```python
from build123d import *

# Parameters (mm, degrees)
F1_DEPTH = 12.7


with BuildPart() as f1:
    # F0 (on Top) → F1 (new body)
    with BuildSketch(Plane.XY):
        with BuildLine():
            ThreePointArc((-26.2838029012, 5.9890534429), (-24.6151248103, 5.9761621536), (-22.9531423273, 6.1260520558))
            ThreePointArc((-22.9531423273, 6.1260520558), (-49.4660776258, 0.5846286719), (-23.509406267, -7.1545136085))
            ThreePointArc((-23.509406267, -7.1545136085), (-25.4282077221, -7.135411063), (-27.3341276607, -7.3581959791))
            ThreePointArc((-27.3341276607, -7.3581959791), (-46.4726203609, 0.8628055089), (-26.2838029012, 5.9890534429))
        make_face()
        with BuildLine():
            Line((-24.5101160102, 0), (-21.5383160102, 0))
            ThreePointArc((-21.5383160102, 0), (-21.8966174323, 3.1436542152), (-22.9531423273, 6.1260520558))
            ThreePointArc((-22.9531423273, 6.1260520558), (-24.6151248103, 5.9761621536), (-26.2838029012, 5.9890534429))
            ThreePointArc((-26.2838029012, 5.9890534429), (-24.9628562451, 3.1230884685), (-24.5101160102, 0))
        make_face()
        with BuildLine():
            ThreePointArc((-23.509406267, -7.1545136085), (-22.0401002948, -3.7105343879), (-21.5383160102, 0))
            Line((-21.5383160102, 0), (-24.5101160102, 0))
            ThreePointArc((-24.5101160102, 0), (-25.2403619408, -3.9407515105), (-27.3341276607, -7.3581959791))
            ThreePointArc((-27.3341276607, -7.3581959791), (-25.4282077221, -7.135411063), (-23.509406267, -7.1545136085))
        make_face()
        with BuildLine():
            ThreePointArc((-13.97, 0), (-9.8782817332, 9.8782817332), (0, 13.97))
            Line((0, 13.97), (0, 21.2281967688))
            ThreePointArc((0, 21.2281967688), (-4.3381640986, 21.9188431605), (-8.2473894167, 23.922494227))
            ThreePointArc((-8.2473894167, 23.922494227), (-12.1416726615, 12.1663301502), (-22.9531423273, 6.1260520558))
            ThreePointArc((-22.9531423273, 6.1260520558), (-21.8966174323, 3.1436542152), (-21.5383160102, 0))
            Line((-21.5383160102, 0), (-13.97, 0))
        make_face()
        with BuildLine():
            Line((0, -16.5764547127), (0, -13.97))
            ThreePointArc((0, -13.97), (-9.8782817332, -9.8782817332), (-13.97, 0))
            Line((-13.97, 0), (-21.5383160102, 0))
            ThreePointArc((-21.5383160102, 0), (-22.0401002948, -3.7105343879), (-23.509406267, -7.1545136085))
            ThreePointArc((-23.509406267, -7.1545136085), (-14.1800112892, -11.2658599468), (-9.5466303459, -20.3473003831))
            ThreePointArc((-9.5466303459, -20.3473003831), (-5.1321883254, -17.5533202567), (0, -16.5764547127))
        make_face()
        with BuildLine():
            ThreePointArc((13.97, -30.5464547127), (12.8498346481, -25.0653371701), (9.6689764472, -20.4632114615))
            ThreePointArc((9.6689764472, -20.4632114615), (9.263305422, -22.3725482488), (9.0618977051, -24.3140865254))
            ThreePointArc((9.0618977051, -24.3140865254), (10.5029749733, -27.2833396443), (10.9982, -30.5464547127))
            ThreePointArc((10.9982, -30.5464547127), (-2.625018329, -41.2267956255), (-9.7451365483, -25.4481494163))
            ThreePointArc((-9.7451365483, -25.4481494163), (-9.4302368554, -22.9061170685), (-9.5466303459, -20.3473003831))
            ThreePointArc((-9.5466303459, -20.3473003831), (-5.5585283155, -43.3629933627), (13.97, -30.5464547127))
        make_face()
        with BuildLine():
            ThreePointArc((9.6689764472, -20.4632114615), (5.2104698339, -17.5845141131), (0, -16.5764547127))
            Line((0, -16.5764547127), (0, -19.5482547127))
            ThreePointArc((0, -19.5482547127), (5.1193540335, -20.8123590938), (9.0618977051, -24.3140865254))
            ThreePointArc((9.0618977051, -24.3140865254), (9.263305422, -22.3725482488), (9.6689764472, -20.4632114615))
        make_face()
        with BuildLine():
            Line((0, -19.5482547127), (0, -16.5764547127))
            ThreePointArc((0, -16.5764547127), (-5.1321883254, -17.5533202567), (-9.5466303459, -20.3473003831))
            ThreePointArc((-9.5466303459, -20.3473003831), (-9.4302368554, -22.9061170685), (-9.7451365483, -25.4481494163))
            ThreePointArc((-9.7451365483, -25.4481494163), (-5.6959732236, -21.1381449668), (0, -19.5482547127))
        make_face()
        with BuildLine():
            Line((23.0888973165, 0), (13.97, 0))
            ThreePointArc((13.97, 0), (9.8782817332, -9.8782817332), (0, -13.97))
            Line((0, -13.97), (0, -16.5764547127))
            ThreePointArc((0, -16.5764547127), (5.2104698339, -17.5845141131), (9.6689764472, -20.4632114615))
            ThreePointArc((9.6689764472, -20.4632114615), (15.2821696202, -11.4178910111), (24.9617009206, -6.9870408157))
            ThreePointArc((24.9617009206, -6.9870408157), (23.5652185436, -3.6168402197), (23.0888973165, 0))
        make_face()
        with BuildLine():
            ThreePointArc((51.0288973165, 0), (41.7222021913, 13.1686934676), (26.2021990138, 8.7916438716))
            ThreePointArc((26.2021990138, 8.7916438716), (28.5955998519, 8.8133611699), (30.9645498306, 9.1552898349))
            ThreePointArc((30.9645498306, 9.1552898349), (42.2518517126, 9.6950310922), (48.0570973165, 0))
            ThreePointArc((48.0570973165, 0), (40.6825557587, -10.3840985518), (28.4485245075, -6.8426517763))
            ThreePointArc((28.4485245075, -6.8426517763), (26.701686584, -6.8321093301), (24.9617009206, -6.9870408157))
            ThreePointArc((24.9617009206, -6.9870408157), (40.6757375362, -13.4936787729), (51.0288973165, 0))
        make_face()
        with BuildLine():
            ThreePointArc((26.2021990138, 8.7916438716), (23.8902038488, 4.6633048748), (23.0888973165, 0))
            Line((23.0888973165, 0), (26.0606973165, 0))
            ThreePointArc((26.0606973165, 0), (27.3638662242, 5.1929543961), (30.9645498306, 9.1552898349))
            ThreePointArc((30.9645498306, 9.1552898349), (28.5955998519, 8.8133611699), (26.2021990138, 8.7916438716))
        make_face()
        with BuildLine():
            Line((26.0606973165, 0), (23.0888973165, 0))
            ThreePointArc((23.0888973165, 0), (23.5652185436, -3.6168402197), (24.9617009206, -6.9870408157))
            ThreePointArc((24.9617009206, -6.9870408157), (26.701686584, -6.8321093301), (28.4485245075, -6.8426517763))
            ThreePointArc((28.4485245075, -6.8426517763), (26.6747987646, -3.6236584423), (26.0606973165, 0))
        make_face()
        with BuildLine():
            ThreePointArc((0, 13.97), (9.8782817332, 9.8782817332), (13.97, 0))
            Line((13.97, 0), (23.0888973165, 0))
            ThreePointArc((23.0888973165, 0), (23.8902038488, 4.6633048748), (26.2021990138, 8.7916438716))
            ThreePointArc((26.2021990138, 8.7916438716), (14.8492633775, 13.7645914435), (9.476547394, 24.9338921412))
            ThreePointArc((9.476547394, 24.9338921412), (5.0876597937, 22.1875619716), (0, 21.2281967688))
            Line((0, 21.2281967688), (0, 13.97))
        make_face()
        with BuildLine():
            ThreePointArc((13.97, 35.1981967688), (-6.3223757342, 47.655663007), (-8.2473894167, 23.922494227))
            ThreePointArc((-8.2473894167, 23.922494227), (-8.7065761615, 27.0814291625), (-9.7451365483, 30.0998914723))
            ThreePointArc((-9.7451365483, 30.0998914723), (-2.625018329, 45.8785376815), (10.9982, 35.1981967688))
            ThreePointArc((10.9982, 35.1981967688), (10.6803409127, 32.5731784398), (9.7451365483, 30.0998914723))
            ThreePointArc((9.7451365483, 30.0998914723), (9.4225906062, 27.5266793177), (9.476547394, 24.9338921412))
            ThreePointArc((9.476547394, 24.9338921412), (12.7974268331, 29.5958074167), (13.97, 35.1981967688))
        make_face()
        with BuildLine():
            Line((0, 24.1999967688), (0, 21.2281967688))
            ThreePointArc((0, 21.2281967688), (5.0876597937, 22.1875619716), (9.476547394, 24.9338921412))
            ThreePointArc((9.476547394, 24.9338921412), (9.4225906062, 27.5266793177), (9.7451365483, 30.0998914723))
            ThreePointArc((9.7451365483, 30.0998914723), (5.6959732236, 25.7898870228), (0, 24.1999967688))
        make_face()
        with BuildLine():
            ThreePointArc((-8.2473894167, 23.922494227), (-4.3381640986, 21.9188431605), (0, 21.2281967688))
            Line((0, 21.2281967688), (0, 24.1999967688))
            ThreePointArc((0, 24.1999967688), (-5.6959732236, 25.7898870228), (-9.7451365483, 30.0998914723))
            ThreePointArc((-9.7451365483, 30.0998914723), (-8.7065761615, 27.0814291625), (-8.2473894167, 23.922494227))
        make_face()
    extrude(amount=F1_DEPTH)


solid = f1.part
```
Could you check a few things on this model? Use its own coordinates, in mm. A direction names the side the tool comes from. Round coordinates to 2 decimals unless told otherwise and drop trailing zeros. Loops run counter-clockwise (first coordinate to the right, second up) from the corner with the lowest first, then second, coordinate; pieces in that order, holes last. Notation, with made-up numbers: M 58.25,88.25 L 66.25,88.25 A22 ccw 66.25,98.25 Z; hole C 68.5,-13.75 d10. An arc over 180 degrees is marked long. Answer as CSV lines item,"result".
1) We'd pull the mould along Y, two halves only. Please class faces 1 (the cylindrical face through (14.98, 13.64, 6.26)), 2 (the flat face through (12, 9, 12.7)), 3 (the cylindrical face through (-49.435, 1.101, 6.261)): released by +Y, released by -Y, zero draft, split by the parting line, or undercut.
From the geometry:
face 1,"undercut"
face 2,"zero draft"
face 3,"split by the parting line"
2) Imagine slicing it at B-B on z = 2.75. List the corners of the cut face in (x, y) for me (1 decimal).
From the geometry:
outline,"M -23.5,-7.2 A15.2 cw -9.5,-20.3 A14 ccw long 9.7,-20.5 A18.4 cw 25,-7 A14 ccw long 26.2,8.8 A17.8 cw 9.5,24.9 A14 ccw long -8.2,23.9 A17.1 cw -23,6.1 A14 ccw long Z; hole C -35.5,0 d22; hole C 0,0 d27.9; hole C 0,-30.5 d22; hole C 0,35.2 d22; hole C 37.1,0 d22"
3) Imagine slicing it at A-A on y = -38.5. List the corners of the cut face in (x, z) for me, and give its area (3 significant figures).
From the geometry:
outline,"M -11.48,0 L -7.6,0 L -7.6,12.7 L -11.48,12.7 Z; M 7.6,0 L 11.48,0 L 11.48,12.7 L 7.6,12.7 Z"
area,"98.8 mm^2"
4) If I drill on probe 1 along Y at (x, z) = (-0.5, 7.75); probe 2 along Y at (x, z) = (-2, 3.5); probe 3 along X at (y, z) = (8, 1.75), over which ranges is the centre line in solid material (lowest first)?
From the geometry:
probe 1,"-44.51 to -41.53, -19.56 to -13.96, 13.96 to 24.21, 46.19 to 49.16"
probe 2,"-44.37 to -41.36, -19.73 to -13.83, 13.83 to 24.38, 46.01 to 49.02"
probe 3,"-46.96 to -43.06, -27.96 to -24.06, -17.22 to -11.45, 11.45 to 29.51, 44.61 to 48.51"
5) Imagine slicing it at C-C on x = -39.5. List the corners of the cut face in (y, z) for me, and give its area (3 significant figures).
From the geometry:
outline,"M -13.39,0 L -10.25,0 L -10.25,12.7 L -13.39,12.7 Z; M 10.25,0 L 13.39,0 L 13.39,12.7 L 10.25,12.7 Z"
area,"79.7 mm^2"
6) For pin 1 Ø6 at (x, y) = (24, -8) entering from +Z; pin 2 Ø3 at (x, z) = (-20.5, 6.5) entering from -Y; pin 3 Ø20 at (x, y) = (0, 35.2) entering from +Z; pin 4 Ø4 at (y, z) = (6.5, 4) entering from +X, each with a flat end and sliding along its axis, tell me the tip position at first contact or that it passes through.
From the geometry:
pin 1,"z = 12.7"
pin 2,"y = -8.19"
pin 3,"through"
pin 4,"x = 50.28"
7) Which directions (+Z, -Z, +X, -X, +Y, -Y) give clear straight access to the entire face, cutting with the end or side of a thin tool? Please do faces 4 (the cylindrical face through (-12.03, 12.3, 6.26)), 5 (the flat face through (12, 9, 0)).
From the geometry:
face 4,"+Z, -Z"
face 5,"-Z, +X, -X, +Y, -Y"
